from build123d import *

# Parameters (mm, degrees)
F0_R      = 19.5
F1_DEPTH  = 7.5
F3_R      = 17.5
F4_DEPTH  = 2
F2_R      = 17.5
F5_DEPTH  = 2
F6_R      = 1.5
F7_DEPTH  = 25
F8_R      = 17.5
F8_R_2    = 2.5
F9_DEPTH  = 4
F10_R     = 17.5
F10_R_2   = 2.5
F11_DEPTH = 4
F12_R     = 20
F12_R_2   = 19.5
F12_R_3   = 17.5
F13_DEPTH = 25
F14_DEPTH = 4


with BuildPart() as f1:
    # F0 (on Right) → F1 (new body, symmetric)
    with BuildSketch(Plane.YZ):
        Circle(F0_R)
    extrude(amount=F1_DEPTH, both=True)

    # F3 (on face) → F4 (cut)
    with BuildSketch(Plane(origin=(-7.5, 0, 0), x_dir=(0, -1, 0), z_dir=(-1, 0, 0))):
        Circle(F3_R)
    extrude(amount=-F4_DEPTH, mode=Mode.SUBTRACT)

    # F2 (on face) → F5 (cut)
    with BuildSketch(Plane.YZ.offset(7.5)):
        Circle(F2_R)
    extrude(amount=-F5_DEPTH, mode=Mode.SUBTRACT)

    # F6 (on face) → F7 (cut)
    with BuildSketch(Plane.YZ.offset(5.5)):
        Circle(F6_R)
    extrude(amount=-F7_DEPTH, mode=Mode.SUBTRACT)

    # F8 (on face) → F9 (cut)
    with BuildSketch(Plane.YZ.offset(5.5)):
        Circle(F8_R)
        Circle(F8_R_2, mode=Mode.SUBTRACT)
    extrude(amount=-F9_DEPTH, mode=Mode.SUBTRACT)

    # F10 (on face) → F11 (cut)
    with BuildSketch(Plane(origin=(-5.5, 0, 0), x_dir=(0, -1, 0), z_dir=(-1, 0, 0))):
        Circle(F10_R)
        Circle(F10_R_2, mode=Mode.SUBTRACT)
    extrude(amount=-F11_DEPTH, mode=Mode.SUBTRACT)

    # F12 (on face) → F13 (cut)
    with BuildSketch(Plane.YZ.offset(7.5)):
        Circle(F12_R)
        Circle(F12_R_2, mode=Mode.SUBTRACT)
        Circle(F12_R_2)
        Circle(F12_R_3, mode=Mode.SUBTRACT)
    extrude(amount=-F13_DEPTH, mode=Mode.SUBTRACT)

    # F14 (cut): a face of the model
    f14_faces = [f1.faces().sort_by_distance(p)[0] for p in [
        (5.5, -2.4292893219, 0),
    ]]
    extrude(f14_faces, amount=-F14_DEPTH, mode=Mode.SUBTRACT)


solid = f1.part
Here's how the part is built. I have some questions about the finished solid (model axes, mm). A direction names the side the tool comes from. Coordinates: 2 decimals unless noted, no trailing zeros. Order: outer loops, then holes, each group sorted by start corner. A loop starts at its lowest first (then second) coordinate and runs counter-clockwise, first axis right, second up. Notation, with made-up numbers: M 73,81.25 L 104,81.25 A31 ccw 104,119.25 Z; hole C 13.25,60 d7. An arc over 180 degrees is marked long. Answer as CSV lines item,"result".
Item 1: If I drill on line 1 (Z direction, x = -3, y = 0); line 2 (Z direction, x = -1.25, y = 0); line 3 (X direction, y = 12, z = 4), over which ranges is the centre line in solid material (lowest first)?
Results found:
line 1,"-2.5 to -1.5, 1.5 to 2.5"
line 2,"-17.5 to -1.5, 1.5 to 17.5"
line 3,"-1.5 to 1.5"
Item 2: Imagine slicing it at C-C on x = 0.25. Write out the boundary of the cut face in (y, z).
Results found:
outline,"C 0,0 d35; hole C 0,0 d3"
Item 3: Imagine slicing it at A-A on y = 0. Write out the boundary of the cut face in (x, z).
Results found:
outline,"M -5.5,-2.5 L -1.5,-2.5 L -1.5,-17.5 L 1.5,-17.5 L 1.5,-1.5 L -5.5,-1.5 Z; M -5.5,1.5 L 1.5,1.5 L 1.5,17.5 L -1.5,17.5 L -1.5,2.5 L -5.5,2.5 Z"
Item 4: On a 3-axis mill with a long thin cutter (end or side, diameter ignored), from which of +Z, -Z, +X, -X, +Y, -Y can I reach the whole of each face in a straight line? I mean faces 4 (the face through (1.5, 0, -4)), 5 (the face through (-3.53, 0.54, -2.44)). Say none if no direction works.
Results found:
face 4,"+Z, -Z, +X, +Y, -Y"
face 5,"-X"
Item 5: Imagine slicing it at D-D on y = 9.5. Write out the boundary of the cut face in (x, z), plus the area to 3 significant figures.
Results found:
outline,"M -1.5,-14.7 L 1.5,-14.7 L 1.5,14.7 L -1.5,14.7 Z"
area,"88.2 mm2"
Item 6: We'd pull the mould along Z, two halves only. Please class faces 1 (the face through (-1.95, -1.5, 0.07)), 2 (the face through (0.021, -13.887, -10.648)), 3 (the face through (-5.5, 0, -2)): +Z half, -Z half, draft (parallel to the pull), parting line (faces both ways), or undercut.
Results found:
face 1,"undercut"
face 2,"parting line"
face 3,"draft"
Item 7: For pin 1 (3 mm diameter, centred on y = -2.5, z = -5, fed in from -X); pin 2 (2 mm diameter, centred on x = -4.5, y = 0.5, fed in from -Z), each with a flat end and sliding along its axis, tell me the tip position at first contact or that it passes through.
Results found:
pin 1,"x = -1.5"
pin 2,"z = -2.5"
